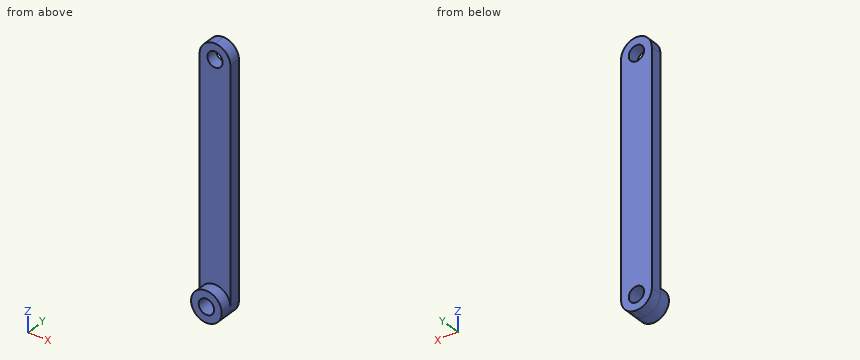
from build123d import *

# Parameters (mm, degrees)
F0_R     = 50.8
F1_DEPTH = 76.2
F2_R     = 101.6
F2_R_2   = 50.8
F3_DEPTH = 76.2


with BuildPart() as f1:
    # F0 (on Front) → F1 (new body)
    with BuildSketch(Plane.XZ):
        with BuildLine():
            Line((-101.6, 1524), (-101.6, 0))
            ThreePointArc((-101.6, 0), (-71.842049, -71.842049), (0, -101.6))
            ThreePointArc((0, -101.6), (71.842049, -71.842049), (101.6, 0))
            Line((101.6, 0), (101.6, 1524))
            ThreePointArc((101.6, 1524), (71.842049, 1595.842049), (0, 1625.6))
            ThreePointArc((0, 1625.6), (-71.842049, 1595.842049), (-101.6, 1524))
        make_face()
        Circle(F0_R, mode=Mode.SUBTRACT)
        with Locations((0, 1524)):
            Circle(F0_R, mode=Mode.SUBTRACT)
    extrude(amount=F1_DEPTH)

    # F2 (on face) → F3 (join)
    with BuildSketch(Plane.XZ.offset(76.2)):
        Circle(F2_R)
        Circle(F2_R_2, mode=Mode.SUBTRACT)
    extrude(amount=F3_DEPTH)


solid = f1.part
Can you work these out from the model? Positions are in its coordinate system, mm. Coordinates: 2 decimals unless noted, no trailing zeros. Loops run counter-clockwise (first coordinate to the right, second up) from the corner with the lowest first, then second, coordinate; pieces in that order, holes last. Notation, with made-up numbers: (-32, 63.5) - (-19, 63.5) arc R24 cw to (-19, 89.5) - close; hole circle Ø10 at (24.25, 17.5). An arc over 180 degrees is marked (long way). Answer as a JSON object with one key per item and string values. Group by question number.
Item 1: If we section it at C-C (z = 1362.5): List the corners of the cut face in (x, y) for me, plus the area to 3 significant figures.
Item 2: If we section it at A-A (y = -20): List the corners of the cut face in (x, z) for me, plus the area to 3 significant figures.
Item 3: If we section it at D-D (y = -94): List the corners of the cut face in (x, z) for me.
Item 4: If we section it at B-B (x = 21): List the corners of the cut face in (y, z) for me.
Item 5: For pin 1 (8 mm diameter, centred on x = -79, z = 529, fed in from -Y); pin 2 (1 mm diameter, centred on x = -6, y = -24, fed in from +Z); pin 3 (6 mm diameter, centred on x = 73, y = -104.5, fed in from +Z), each with a flat end and sliding along its axis, tell me the tip position at first contact or that it passes through.
Item 6: If I drill on L1, parallel to Z at x = 2, y = -27; L2, parallel to Z at x = 0, y = -105; L3, parallel to Z at x = -22, y = -50, over which ranges is the centre line in solid material (lowest first)? Write a range as from..to.
Returned:
{
 "1": {"outline": "(-101.6, -76.2) - (101.6, -76.2) - (101.6, 0) - (-101.6, 0) - close", "area": "15,500 mm²"},
 "2": {"outline": "(-101.6, 0) arc R101.6 ccw to (101.6, 0) - (101.6, 1524) arc R101.6 ccw to (-101.6, 1524) - close; hole circle Ø101.6 at (0, 0); hole circle Ø101.6 at (0, 1524)", "area": "326,000 mm²"},
 "3": {"outline": "circle Ø203.2 at (0, 0); hole circle Ø101.6 at (0, 0)"},
 "4": {"outline": "(-152.4, -99.41) - (0, -99.41) - (0, -46.26) - (-152.4, -46.26) - close; (-152.4, 46.26) - (0, 46.26) - (0, 1477.74) - (-76.2, 1477.74) - (-76.2, 99.41) - (-152.4, 99.41) - close; (-76.2, 1570.26) - (0, 1570.26) - (0, 1623.41) - (-76.2, 1623.41) - close"},
 "5": {"pin 1": "stops at y = -76.2", "pin 2": "stops at z = 1625.45", "pin 3": "stops at z = 73.64"},
 "6": {"L1": "z = -101.58..-50.76, 50.76..1473.24, 1574.76..1625.58", "L2": "z = -101.6..-50.8, 50.8..101.6", "L3": "z = -99.19..-45.79, 45.79..1478.21, 1569.79..1623.19"}
}
